Source: CAD feature listing. Evaluate the final solid. Frame: model axes, mm. A direction names the side the tool comes from. Coordinates: 2 decimals unless noted, no trailing zeros. Loops run counter-clockwise (first coordinate to the right, second up) from the corner with the lowest first, then second, coordinate; pieces in that order, holes last.
from build123d import *

# Parameters (mm, degrees)
SKETCH1_W                = 136
SKETCH1_H                = 122
BOSS_EXTRUDE1_DEPTH      = 26
FILLET1_R                = 20
SHELL1_T                 = -4
SHELL1_THICKNESS_2_DEPTH = 1
CUT_EXTRUDE1_REACH       = 96.202
SKETCH2_W                = 113
SKETCH2_H                = 77
FILLET2_R                = 4
M3_CLEARANCE_HOLE1_D     = 3.4
CUT_EXTRUDE2_DEPTH       = 4
BOSS_EXTRUDE3_DEPTH      = 56.25


with BuildPart() as part:
    # Sketch1 → Boss-Extrude1 (new body)
    with BuildSketch(Plane(origin=(0, 0, 0), x_dir=(1, 0, 0), z_dir=(0, 1, 0))):
        Rectangle(SKETCH1_W, SKETCH1_H)
    extrude(amount=BOSS_EXTRUDE1_DEPTH)

    # Fillet1
    fillet1_edges = [part.edges().sort_by_distance(p)[0] for p in [
        (68, 13, 61),
        (-68, 13, 61),
        (-68, 13, -61),
        (68, 13, -61),
    ]]
    fillet(fillet1_edges, radius=FILLET1_R)

    # Shell1
    shell1_openings = [part.faces().sort_by_distance(p)[0] for p in [
        (0, 26, 0),
    ]]
    offset(amount=SHELL1_T, openings=shell1_openings, kind=Kind.INTERSECTION)

    # Shell1 thickness 2 face (on inner face of the shell) → Shell1 thickness 2 (cut)
    with BuildSketch(Plane(origin=(0, 4, 0), x_dir=(0, 0, -1), z_dir=(0, -1, 0))):
        with BuildLine():
            ThreePointArc((57, -48), (52.313708499, -59.313708499), (41, -64))
            Line((41, -64), (-41, -64))
            ThreePointArc((-41, -64), (-52.313708499, -59.313708499), (-57, -48))
            Line((-57, -48), (-57, 48))
            ThreePointArc((-57, 48), (-52.313708499, 59.313708499), (-41, 64))
            Line((-41, 64), (41, 64))
            ThreePointArc((41, 64), (52.313708499, 59.313708499), (57, 48))
            Line((57, 48), (57, -48))
        make_face()
    extrude(amount=SHELL1_THICKNESS_2_DEPTH, mode=Mode.SUBTRACT)

    # Sketch2 → Cut-Extrude1 (cut, up to next)
    with BuildSketch(Plane(origin=(0, 3, 0), x_dir=(1, 0, 0), z_dir=(0, 1, 0)), mode=Mode.PRIVATE) as cut_extrude1_sk1:
        Rectangle(SKETCH2_W, SKETCH2_H)
    cut_extrude1_tool1 = extrude(cut_extrude1_sk1.sketch, amount=-CUT_EXTRUDE1_REACH, mode=Mode.PRIVATE) & part.part
    add(cut_extrude1_tool1.solids().sort_by_distance((0, 3, 0))[0], mode=Mode.SUBTRACT)

    # Fillet2
    fillet2_edges = [part.edges().sort_by_distance(p)[0] for p in [
        (56.5, 1.5, -38.5),
        (56.5, 1.5, 38.5),
        (-56.5, 1.5, 38.5),
        (-56.5, 1.5, -38.5),
    ]]
    fillet(fillet2_edges, radius=FILLET2_R)

    # M3 Clearance Hole1 (through all)
    with Locations(Plane(origin=(0, 3, 0), x_dir=(1, 0, 0), z_dir=(0, 1, 0))):
        with Locations((-59, 39), (59, 39), (59, -39), (-59, -39)):
            Hole(M3_CLEARANCE_HOLE1_D / 2)

    # Sketch5 → Cut-Extrude2 (cut)
    with BuildSketch(Plane(origin=(0, 26, 0), x_dir=(1, 0, 0), z_dir=(0, 1, 0))):
        with BuildLine():
            Line((-68, 41), (-68, -41))
            ThreePointArc((-68, -41), (-62.142135624, -55.142135624), (-48, -61))
            Line((-48, -61), (48, -61))
            ThreePointArc((48, -61), (62.142135624, -55.142135624), (68, -41))
            Line((68, -41), (68, 41))
            ThreePointArc((68, 41), (62.142135624, 55.142135624), (48, 61))
            Line((48, 61), (41.5, 61))
            Line((41.5, 61), (41.5, 59))
            Line((41.5, 59), (48, 59))
            ThreePointArc((48, 59), (60.727922061, 53.727922061), (66, 41))
            Line((66, 41), (66, -41))
            ThreePointArc((66, -41), (60.727922061, -53.727922061), (48, -59))
            Line((48, -59), (-48, -59))
            ThreePointArc((-48, -59), (-60.727922061, -53.727922061), (-66, -41))
            Line((-66, -41), (-66, 41))
            ThreePointArc((-66, 41), (-60.727922061, 53.727922061), (-48, 59))
            Line((-48, 59), (-41.5, 59))
            Line((-41.5, 59), (-41.5, 61))
            Line((-41.5, 61), (-48, 61))
            ThreePointArc((-48, 61), (-62.142135624, 55.142135624), (-68, 41))
        make_face()
    extrude(amount=-CUT_EXTRUDE2_DEPTH, mode=Mode.SUBTRACT)

    # Sketch9 → Boss-Extrude3 (add)
    with BuildSketch(Plane(origin=(0, 26, 0), x_dir=(1, 0, 0), z_dir=(0, 1, 0))):
        Polygon((-41.5, 61), (-41.5, 59), (-45.5, 59), (-45.5, 57), (45.5, 57), (45.5, 59), (41.5, 59), (41.5, 61), align=None)
    extrude(amount=BOSS_EXTRUDE3_DEPTH)


solid = part.part
Q1. Section B-B, the plane y = 6.5. Return the cut outline in (x, z), plus the area to 3 significant figures.
Q2. Access query for faces 1 (the cylindrical face through (-55.359, 1.479, -37.297)), 2 (the cylindrical face through (-60.587, 24.028, 53.867)), 3 (the flat face through (-66, 24, 1)), 4 (the flat face through (-51, 22, -59)), 5 (the flat face through (66, 24, -1)). Directions: +Z, -Z, +X, -X, +Y, -Y. A direction counts if a zero-diameter tool reaches every point of the face in a straight line with its end or side. Return the directions, or none.
Q3. Line query: line 1 along Z through (x, y) = (10.5, 22.5); line 2 along Z through (x, y) = (-59, 0.8); line 3 along Z through (x, y) = (38, 9). Output: solid intervals per line, ascending.
Q4. Section C-C, the plane x = -59. Return the cut outline in (y, z), plus the area to 3 significant figures.
Q5. Draft query along X for faces 6 (the cylindrical face through (-57.65, 1.48, -37.97)), 7 (the cylindrical face through (60.587, 24.028, -53.867)), 8 (the flat face through (-1, 14, 57)), 9 (the flat face through (-1, 11, 61)). Return one class per face: +X half, -X half, draft (parallel to the pull), parting line (faces both ways), or undercut.
Q6. Contact query for flat-ended pins moving along their axis: pin 1 Ø2 at (y, z) = (50.5, -58) entering from -X; pin 2 Ø5 at (x, z) = (-50, -46) entering from +Y; pin 3 Ø3 at (x, y) = (10, 24.5) entering from +Z; pin 4 Ø2 at (x, z) = (59, -39) entering from -Y. Output: stop coordinate, or through.
Q7. Section D-D, the plane y = 36. Return the cut outline in (x, z), plus the area to 3 significant figures.
Q8. Section A-A, the plane x = -11. Return the cut outline in (y, z).
Derived:
1. outline: (-68, -41) arc R20 ccw to (-48, -61) - (48, -61) arc R20 ccw to (68, -41) - (68, 41) arc R20 ccw to (48, 61) - (-48, 61) arc R20 ccw to (-68, 41) - close; hole (-64, -41) arc R16 ccw to (-48, -57) - (48, -57) arc R16 ccw to (64, -41) - (64, 41) arc R16 ccw to (48, 57) - (-48, 57) arc R16 ccw to (-64, 41) - close
1. area: 1,880 mm2
2. face 1: +Y, -Y
2. face 2: +Z, -X, +Y
2. face 3: +Z, -Z, -X, +Y
2. face 4: +Y
2. face 5: +Z, -Z, +X, +Y
3. line 1: z = -61 to -57, 57 to 59
3. line 2: z = -57.7 to -40.7, -37.3 to 37.3, 40.7 to 57.7
3. line 3: z = -61 to -57, 57 to 61
4. outline: (0, -57.7) - (22, -57.7) - (22, -55.25) - (26, -55.25) - (26, -52.62) - (3, -52.62) - (3, -40.7) - (0, -40.7) - close; (0, -37.3) - (3, -37.3) - (3, 37.3) - (0, 37.3) - close; (0, 40.7) - (3, 40.7) - (3, 52.62) - (26, 52.62) - (26, 55.25) - (22, 55.25) - (22, 57.7) - (0, 57.7) - close
4. area: 540 mm2
5. face 6: undercut
5. face 7: +X half
5. face 8: undercut
5. face 9: draft
6. pin 1: stops at x = -45.5
6. pin 2: stops at y = 3
6. pin 3: stops at z = 59
6. pin 4: passes through
7. outline: (-45.5, -59) - (-41.5, -59) - (-41.5, -61) - (41.5, -61) - (41.5, -59) - (45.5, -59) - (45.5, -57) - (-45.5, -57) - close
7. area: 348 mm2
8. outline: (0, -61) - (82.25, -61) - (82.25, -57) - (3, -57) - (3, -38.5) - (0, -38.5) - close; (0, 38.5) - (3, 38.5) - (3, 57) - (26, 57) - (26, 59) - (22, 59) - (22, 61) - (0, 61) - close
